Design review of the part built by this model. Coordinates are the model's own, in mm. Face numbers are marked on the shaded views. A direction names the side the tool comes from. Coordinates: 2 decimals unless noted, no trailing zeros. Write each loop counter-clockwise with the first axis right and the second up, starting at its lowest first coordinate (ties: lowest second). Pieces come first, ordered by that corner, then holes. Notation, with made-up numbers: (83, 24.5) - (102, 24.5) arc R19 ccw to (102, 51.5) - close; hole circle Ø6 at (66, 11). An arc over 180 degrees is marked (long way). One line per item, written item: value.
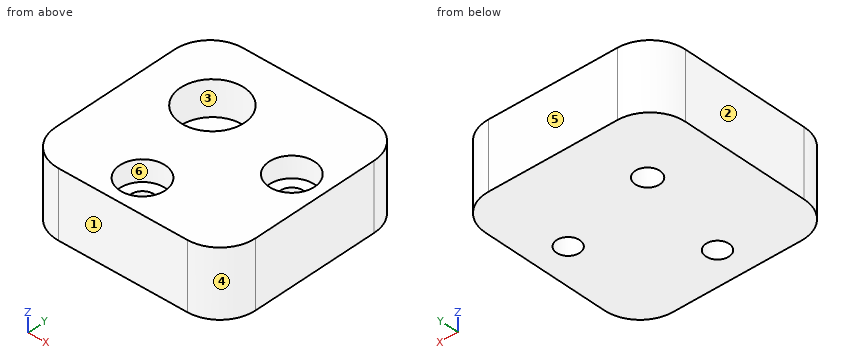
from build123d import *

# Parameters (mm, degrees)
F0_W           = 28.575
F0_H           = 28.575
F1_DEPTH       = 9.525
F3_D           = 3.3
F3_CBORE_D     = 6.5
F3_CBORE_DEPTH = 3
F4_R           = 4.55
F5_DEPTH       = 5
F6_R           = 1.7526
F7_DEPTH       = 4.526
F8_R           = 5.08


with BuildPart() as f1:
    # F0 (on Top) → F1 (new body)
    with BuildSketch(Plane.XY):
        with Locations((-14.2875, 14.2875)):
            Rectangle(F0_W, F0_H)
    extrude(amount=F1_DEPTH)

    # F3 (through all)
    with Locations(Plane.XY.offset(9.525)):
        with Locations((-15.875, 4.7625), (-4.7625, 15.875)):
            CounterBoreHole(F3_D / 2, F3_CBORE_D / 2, F3_CBORE_DEPTH)

    # F4 (on face) → F5 (cut)
    with BuildSketch(Plane.XY.offset(9.525)):
        with Locations((-19.05, 19.05)):
            Circle(F4_R)
    extrude(amount=-F5_DEPTH, mode=Mode.SUBTRACT)

    # F6 (on face) → F7 (cut, through all)
    with BuildSketch(Plane.XY.offset(4.525)):
        with Locations((-19.05, 19.05)):
            Circle(F6_R)
    extrude(amount=-F7_DEPTH, mode=Mode.SUBTRACT)

    # F8
    f8_edges = [f1.edges().sort_by_distance(p)[0] for p in [
        (0, 0, 4.7625),
        (-28.575, 0, 4.7625),
        (-28.575, 28.575, 4.7625),
        (0, 28.575, 4.7625),
    ]]
    fillet(f8_edges, radius=F8_R)


solid = f1.part
1. Insertion check: pin 1 Ø5.5 at (x, y) = (-15.88, 4.76) entering from -Z; pin 2 Ø4.5 at (x, y) = (-4.76, 15.88) entering from +Z (3 decimals); pin 3 Ø3 at (x, y) = (-19.05, 19.05) entering from -Z; pin 4 Ø4.5 at (x, y) = (-20.5, 18.5) entering from +Z (3 decimals). Each pin has a flat end and moves straight along its axis. Give the tip position at first contact, or say it passes through.
Answer block:
pin 1: stops at z = 0
pin 2: stops at z = 6.525
pin 3: passes through
pin 4: stops at z = 4.525
2. Consider section C-C, the plane x = -7.5. Write out the cut boundary in (y, z) (3 decimals), then the cut area to 3 significant figures.
Answer block:
outline: (0, 0) - (28.575, 0) - (28.575, 9.525) - (17.627, 9.525) - (17.627, 6.525) - (14.123, 6.525) - (14.123, 9.525) - (0, 9.525) - close
area: 262 mm^2
3. Consider section B-B, the plane z = 5.25. Give the number of separate pieces and of enclosed holes in the cut face, then the cut area to 3 significant figures.
Answer block:
separate pieces: 1
enclosed holes: 3
area: 712 mm^2
4. Wall thickness on line 1 along Y through (x, z) = (-19.05, 2.4) (3 decimals); line 2 along X through (y, z) = (15.25, 7) (1 decimal); line 3 along Z through (x, y) = (-5.5, 13) (3 decimals): over which ranges is each line inside the solid? List them lowest first.
Answer block:
line 1: y = 0 to 17.297, 20.803 to 28.575
line 2: x = -28.6 to -21.6, -16.5 to -8, -1.6 to 0
line 3: z = 0 to 6.525
5. For the marked faces 5 and 6, list the 3-axis set-ups (+Z, -Z, +X, -X, +Y, -Y) from which the entire face can be reached by the end or side of a thin tool; tool diameter is ignored.
Answer block:
face 5: +Z, -Z, +X, -X, +Y
face 6: +Z
6. Consider section D-D, the plane y = 20. Write out the cut boundary in (x, z) (3 decimals), then the cut area to 3 significant figures.
Answer block:
outline: (-28.575, 0) - (-20.523, 0) - (-20.523, 4.525) - (-23.5, 4.525) - (-23.5, 9.525) - (-28.575, 9.525) - close; (-17.577, 0) - (0, 0) - (0, 9.525) - (-14.6, 9.525) - (-14.6, 4.525) - (-17.577, 4.525) - close
area: 214 mm^2
7. Mouldability with a two-part tool opening along X and no side actions: class the marked faces 1, 2, 3 and 4 as released by +X, released by -X, zero draft, split by the parting line, or undercut.
Answer block:
face 1: zero draft
face 2: released by -X
face 3: undercut
face 4: released by +X
8. Consider section A-A, the plane y = 5.75. Write out the cut boundary in (x, z) (3 decimals), then the cut area to 3 significant figures.
Answer block:
outline: (-28.575, 0) - (-17.197, 0) - (-17.197, 6.525) - (-18.971, 6.525) - (-18.971, 9.525) - (-28.575, 9.525) - close; (-14.553, 0) - (0, 0) - (0, 9.525) - (-12.779, 9.525) - (-12.779, 6.525) - (-14.553, 6.525) - close
area: 236 mm^2
